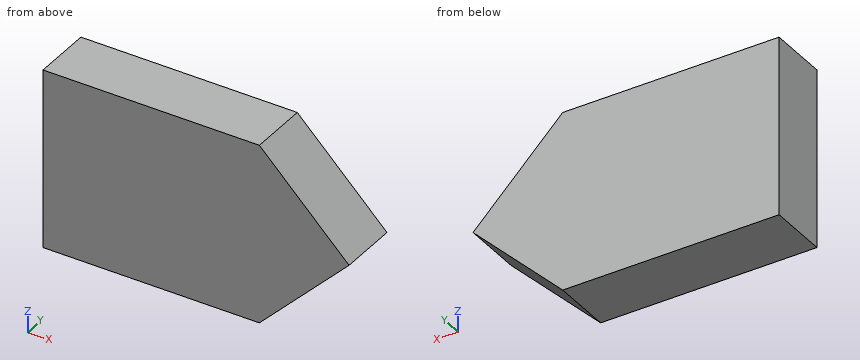
from build123d import *

# Parameters (mm, degrees)
SKETCH1_W           = 91.9
SKETCH1_H           = 38.1
BOSS_EXTRUDE1_DEPTH = 25.4


with BuildPart() as part:
    # Sketch1 → Boss-Extrude1 (new body)
    with BuildSketch(Plane(origin=(0, 0, 0), x_dir=(1, 0, 0), z_dir=(0, 1, 0))):
        with Locations((45.95, 19.05)):
            Rectangle(SKETCH1_W, SKETCH1_H)
        Polygon((91.9, 0), (130, 38.1), (91.9, 38.1), align=None)
        Polygon((130, 38.1), (91.9, 76.2), (91.9, 38.1), align=None)
        with Locations((45.95, 57.15)):
            Rectangle(SKETCH1_W, SKETCH1_H)
    extrude(amount=BOSS_EXTRUDE1_DEPTH)


solid = part.part
The listing builds one solid part. Answer for the finished solid, in the listing's coordinates (mm). Coordinates: 2 decimals unless noted, no trailing zeros. Write each loop counter-clockwise with the first axis right and the second up, starting at its lowest first coordinate (ties: lowest second). Pieces come first, ordered by that corner, then holes. Notation, with made-up numbers: (57, 27.5) - (66, 27.5) arc R24 ccw to (66, 59.5) - close; hole circle Ø4 at (30.5, 1). An arc over 180 degrees is marked (long way). Return JSON: item names as keys, results as strings.
1. The part is cut by section B-B on y = 11.5. Determine the outline of the cut face in (x, z).
Final values:
{"outline": "(0, -76.2) - (91.9, -76.2) - (130, -38.1) - (91.9, 0) - (0, 0) - close"}
2. The part is cut by section C-C on x = 121. Determine the outline of the cut face in (y, z), then the cut area to 3 significant figures.
Final values:
{"outline": "(0, -47.1) - (25.4, -47.1) - (25.4, -29.1) - (0, -29.1) - close", "area": "457 mm^2"}
3. Consider line 1 along X through (y, z) = (6.75, -13); line 2 along X through (y, z) = (23.75, -49); line 3 along Z through (x, y) = (113, 6.25). Determine where each line is inside the solid, lowest interval first.
Final values:
{"line 1": "0 to 104.9", "line 2": "0 to 119.1", "line 3": "-55.1 to -21.1"}
4. The part is cut by section A-A on z = -24. Determine the outline of the cut face in (x, y).
Final values:
{"outline": "(0, 0) - (115.9, 0) - (115.9, 25.4) - (0, 25.4) - close"}
5. Each of these flat-tipped pins is pushed along its axis until it touches: pin 1 Ø1.5 at (y, z) = (18, -19.5) entering from +X; pin 2 Ø8 at (x, y) = (104.5, 11) entering from +Z. Where does it stop, or does it pass through?
Final values:
{"pin 1": "x = 112.15", "pin 2": "z = -8.6"}
